Answer from the drawing. Dimensions are ordinates in mm from the lowest x, y and z of the part. Give positions to 0.01 mm unless a question says otherwise; leave off trailing zeros. Write each loop counter-clockwise with the first axis right and the second up, starting at its lowest first coordinate (ties: lowest second). Pieces come first, ordered by that corner, then holes. Notation, with made-up numbers: M -34.75,-22.75 L -7.75,-22.75 A29 ccw -7.75,-1.75 Z; hole C 22.25,79 d2. An arc over 180 degrees is marked long. Write each question's results on one line, items separated by ' | '. Start each with the question number.
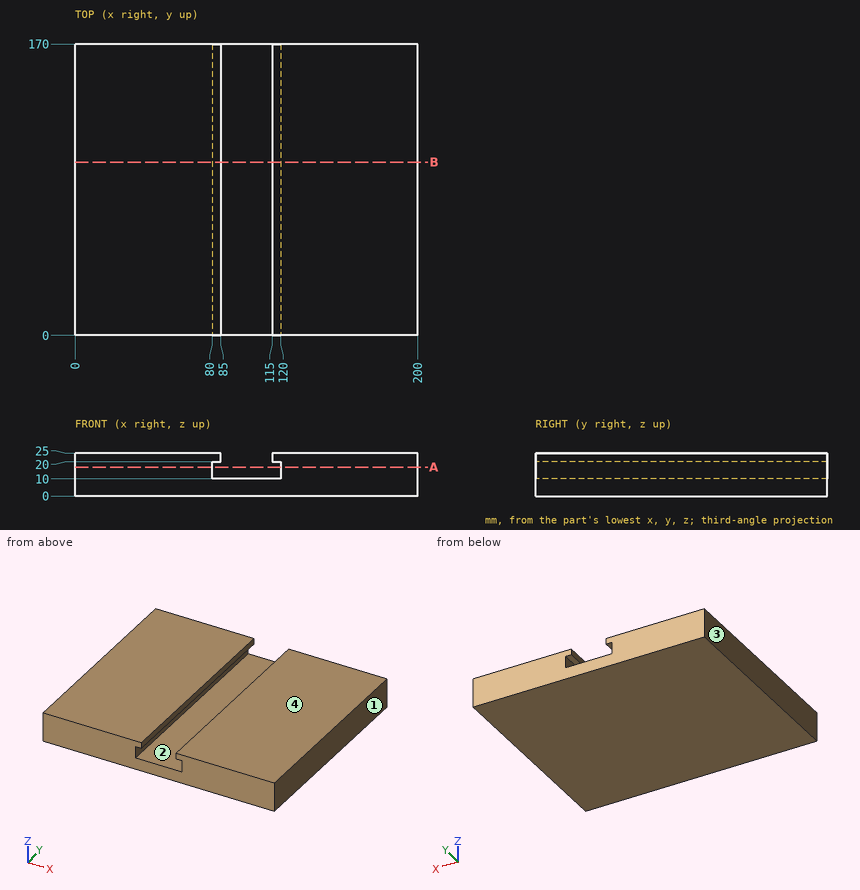
Item 1: Section A-A, the plane z = 17 is taken. Determine the outline of the cut face in (x, y).
Item 2: Determine the mould class of the marked faces 1, 2, 3 and 4 for opening direction X: +X half, -X half, draft (parallel to the pull), parting line (faces both ways), or undercut.
Item 3: Straight lines are drawn through the part: line 1 (X direction, y = 92, z = 18.75); line 2 (Z direction, x = 119, y = 144.5); line 3 (Z direction, x = 96, y = 70). For each, find the intervals that lie inside material, in ascending order.
Item 4: Section B-B, the plane y = 101 is taken. Determine the outline of the cut face in (x, z).
Worked out:
1) outline: M 0,0 L 80,0 L 80,170 L 0,170 Z; M 120,0 L 200,0 L 200,170 L 120,170 Z
2) face 1: +X half | face 2: undercut | face 3: -X half | face 4: draft
3) line 1: x = 0 to 80, 120 to 200 | line 2: z = 0 to 10, 20 to 25 | line 3: z = 0 to 10
4) outline: M 0,0 L 200,0 L 200,25 L 115,25 L 115,20 L 120,20 L 120,10 L 80,10 L 80,20 L 85,20 L 85,25 L 0,25 Z
